from build123d import *

# Parameters (mm, degrees)
F1_DEPTH = 19.05


with BuildPart() as f1:
    # F0 (on Front) → F1 (new body)
    with BuildSketch(Plane.XZ):
        Polygon((17.768437, 18.246084), (0, 0), (0, -3.72564), (17.768437, 14.424915), align=None)
    extrude(amount=F1_DEPTH)


with BuildPart() as f2_1:
    # F2: copy of F1
    add(f1.part)


solid = f1.part
The listing builds one solid part. Answer for the finished solid, in the listing's coordinates (mm). Give positions to 0.01 mm unless a question says otherwise; leave off trailing zeros. Write each loop counter-clockwise with the first axis right and the second up, starting at its lowest first coordinate (ties: lowest second). Pieces come first, ordered by that corner, then holes. Notation, with made-up numbers: (-21.5, 53) - (-16.5, 53) arc R27 cw to (-16.5, 77) - close; hole circle Ø2 at (-10, -2). An arc over 180 degrees is marked (long way). One line per question, with ' | ' between items. Start each with the question number.
1. Given P1, Ø1, axis at x = 4, y = -6, coming from the +Z side; P2, Ø8, axis at y = -15.5, z = 5.5, coming from the -X side; P3, Ø6, axis at y = -10.5, z = 4.5, coming from the +X side, each flat-ended and moving along its own axis, determine where each tip first touches the part or whether it passes through.
2. Straight lines are drawn through the part: line 1 (Z direction, x = 16, y = -7.75); line 2 (Z direction, x = 15.5, y = -12); line 3 (X direction, y = -13.5, z = 9.75). For each, find the intervals that lie inside material, in ascending order.
3. Section B-B, the plane x = 5.75 is taken. Determine the outline of the cut face in (y, z), then the cut area to 3 significant figures.
4. Section A-A, the plane y = -15.5 is taken. Determine the outline of the cut face in (x, z).
5. Determine the mould class of faces 1 (the face through (8.76, -9.39, 5.22)), 2 (the face through (9, -19.05, 7)), 3 (the face through (9, 0, 7)) for opening direction Y: +Y half, -Y half, draft (parallel to the pull), parting line (faces both ways), or undercut.
Result:
1) P1: stops at z = 4.62 | P2: stops at x = 1.46 | P3: stops at x = 10.99
2) line 1: z = 12.62 to 16.43 | line 2: z = 12.11 to 15.92 | line 3: x = 9.49 to 13.19
3) outline: (-19.05, 2.15) - (0, 2.15) - (0, 5.9) - (-19.05, 5.9) - close | area: 71.6 mm2
4) outline: (0, -3.73) - (17.77, 14.42) - (17.77, 18.25) - (0, 0) - close
5) face 1: draft | face 2: -Y half | face 3: +Y half
